```python
from build123d import *

# Parameters (mm, degrees)
SKETCH1_R                  = 26.8
MAIN_BODY_EXTRUDE_DEPTH    = 43.52
ANGLED_EXTRUDE_OUTLINE_R   = 26.8
ANGLED_EXTRUDE_DEPTH       = 5.63358701
ANGLED_START               = 46.082955702
ANGLED_EXTRUDE_2_OUTLINE_W = 57
ANGLED_EXTRUDE_2_OUTLINE_H = 56
ANGLED_EXTRUDE_2_DEPTH     = 6.917044298
SKETCH8_R                  = 16.325
ATTACHMENT_EXTRUDE_DEPTH   = 22.5
SKETCH11_R                 = 12.7625
SKETCH11_R_2               = 11.2625
TUBING_HOLE_DEPTH          = 45
SKETCH13_R                 = 2
BOLT_HOLE_DEPTH            = 25
SKETCH14_W                 = 34.35
SKETCH14_H                 = 34.35
CUT_EXTRUDE3_DEPTH         = 4
SKETCH16_W                 = 23.74
SKETCH16_H                 = 28.35
CUT_EXTRUDE5_DEPTH         = 1
FILLET3_R                  = 5
SKETCH18_R                 = 16.824719049
CUT_EXTRUDE6_DEPTH         = 5


with BuildPart() as part:
    # Sketch1 → Main Body Extrude (new body)
    with BuildSketch(Plane(origin=(0, 0, 0), x_dir=(1, 0, 0), z_dir=(0, 1, 0))):
        with Locations(Location((0, 0, 0), (0, 0, 270))):
            Circle(SKETCH1_R)
    extrude(amount=MAIN_BODY_EXTRUDE_DEPTH)

    # Angled Extrude: read off the stored shape, not the designer's step
    # Angled Extrude outline → Angled Extrude (add)
    with BuildSketch(Plane(origin=(0, 43.52, 0), x_dir=(1, 0, 0), z_dir=(0, 1, 0))):
        Circle(ANGLED_EXTRUDE_OUTLINE_R)
    extrude(amount=ANGLED_EXTRUDE_DEPTH)

    # Angled Extrude 2 outline → Angled Extrude 2 (cut)
    with BuildSketch(Plane(origin=(0, 0, 0), x_dir=(0.9945218953682733, -0.10452846326765303, 0), z_dir=(0.10452846326765304, 0.9945218953682734, 0)).offset(ANGLED_START)):
        with Locations((-4.5, 0)):
            Rectangle(ANGLED_EXTRUDE_2_OUTLINE_W, ANGLED_EXTRUDE_2_OUTLINE_H)
    extrude(amount=ANGLED_EXTRUDE_2_DEPTH, mode=Mode.SUBTRACT)

    # Sketch8 → Attachment Extrude (add)
    with BuildSketch(Plane(origin=(4.816980542, 45.830508449, 0), x_dir=(0.9945218953682734, -0.10452846326765328, 0), z_dir=(0.10452846326765328, 0.9945218953682734, 0))):
        with Locations((-2.478668524, 0)):
            Circle(SKETCH8_R)
    extrude(amount=ATTACHMENT_EXTRUDE_DEPTH)

    # Sketch11 → Tubing Hole (cut)
    with BuildSketch(Plane(origin=(7.168870966, 68.207251095, 0), x_dir=(0.9945218953682734, -0.10452846326765329, 0), z_dir=(0.10452846326765329, 0.9945218953682734, 0))):
        with Locations(Location((-2.478668524, 0, 0), (0, 0, 180))):
            Circle(SKETCH11_R)
        with Locations(Location((-2.478668524, 0, 0), (0, 0, 180))):
            Circle(SKETCH11_R_2, mode=Mode.SUBTRACT)
    extrude(amount=-TUBING_HOLE_DEPTH, mode=Mode.SUBTRACT)

    # Sketch13 → Bolt Hole (cut, symmetric)
    with BuildSketch(Plane.XY):
        with Locations((3.397175056, 56.034818814)):
            Circle(SKETCH13_R)
    extrude(amount=BOLT_HOLE_DEPTH, both=True, mode=Mode.SUBTRACT)

    # Sketch14 → Cut-Extrude3 (cut)
    with BuildSketch(Plane.XZ):
        Rectangle(SKETCH14_W, SKETCH14_H)
    extrude(amount=-CUT_EXTRUDE3_DEPTH, mode=Mode.SUBTRACT)

    # Sketch16 → Cut-Extrude5 (cut)
    with BuildSketch(Plane.XZ.offset(-4)):
        with Locations((-2.305, 0)):
            Rectangle(SKETCH16_W, SKETCH16_H)
    extrude(amount=-CUT_EXTRUDE5_DEPTH, mode=Mode.SUBTRACT)

    # Fillet1: read off the stored shape, not the designer's step
    # Fillet1 outline → Fillet1 (revolve, cut)
    with BuildSketch(Plane.XY):
        with BuildLine():
            ThreePointArc((26.8, 2), (26.214213562, 0.585786438), (24.8, 0))
            Line((24.8, 0), (26.8, 0))
            Line((26.8, 0), (26.8, 2))
        make_face()
    revolve(axis=Axis((0, 0, 0), (0, 1, 0)), mode=Mode.SUBTRACT)

    # Fillet3
    fillet3_edges = [part.edges().sort_by_distance(p)[0] for p in [
        (-13.883679518, 47.796027024, 0),
    ]]
    fillet(fillet3_edges, radius=FILLET3_R)

    # Sketch18 → Cut-Extrude6 (cut)
    with BuildSketch(Plane(origin=(7.168870966, 68.207251095, 0), x_dir=(0.9945218953682734, -0.10452846326765328, 0), z_dir=(0.10452846326765328, 0.9945218953682734, 0))):
        with Locations((-2.478668524, 0)):
            Circle(SKETCH18_R)
    extrude(amount=-CUT_EXTRUDE6_DEPTH, mode=Mode.SUBTRACT)


solid = part.part
```
Source: CAD feature listing. Evaluate the final solid. Frame: model axes, mm. A direction names the side the tool comes from. Coordinates: 2 decimals unless noted, no trailing zeros. Use a Markdown table: item, result. Add a question column.
Q1. Material intervals for L1, parallel to X at y = 53.5, z = 9; L2, parallel to Z at x = 2, y = 49.5; L3, parallel to X at y = 60, z = 8, sorted ascending.
Q2. Access query for faces 4 (the flat face through (-2, 5, 0)), 5 (the flat face through (-6.52, 24.4, -9.39)), 6 (the cylindrical face through (9.974, 25.247, 24.875)). Directions: +Z, -Z, +X, -X, +Y, -Y. A direction counts if a zero-diameter tool reaches every point of the face in a straight line with its end or side. Return the directions, or none.
Q3. First-contact query: pin 1 (3 mm diameter, centred on y = 1, z = -6, fed in from -X); pin 2 (6 mm diameter, centred on y = 9.5, z = -4, fed in from +X); pin 3 (2 mm diameter, centred on x = 1.5, z = 21, fed in from +Y); pin 4 (3 mm diameter, centred on x = 3.4, y = 56.03, fed in from -Z). Flat tips, straight axial feed; report the tip coordinate or a pass-through.
Q4. Section query A-A, the plane y = 50.5. State how many separate pieces and enclosed holes the cut face has, and give its area (3 significant figures).
Q5. Draft query along Y for faces 1 (the flat face through (17.175, 2, 0)), 2 (the flat face through (-17.992, 48.228, -8.066)), 3 (the cylindrical face through (-3.05, 44.42, -9.99)). Return one class per face: pulls with the +Y half, pulls with the -Y half, needs draft (parallel to the pull), parting line crosses it, or undercut.
Result:
| question | item | result |
|---|---|---|
| 1 | L1 | x = -10.56 to -5.97, -3.68 to 9.94, 12.23 to 16.83 |
| 1 | L2 | z = -16.59 to -12.74, -11.24 to 11.24, 12.74 to 16.59 |
| 1 | L3 | x = -10.49 to -6.18, -4.16 to 11.79, 13.81 to 18.12 |
| 2 | face 4 | -Y |
| 2 | face 5 | none |
| 2 | face 6 | +Y, -Y |
| 3 | pin 1 | stops at x = -26.37 |
| 3 | pin 2 | stops at x = 26.78 |
| 3 | pin 3 | stops at y = 46.37 |
| 3 | pin 4 | passes through |
| 4 | separate pieces | 2 |
| 4 | enclosed holes | 1 |
| 4 | area | 745 mm2 |
| 5 | face 1 | needs draft |
| 5 | face 2 | pulls with the +Y half |
| 5 | face 3 | undercut |
